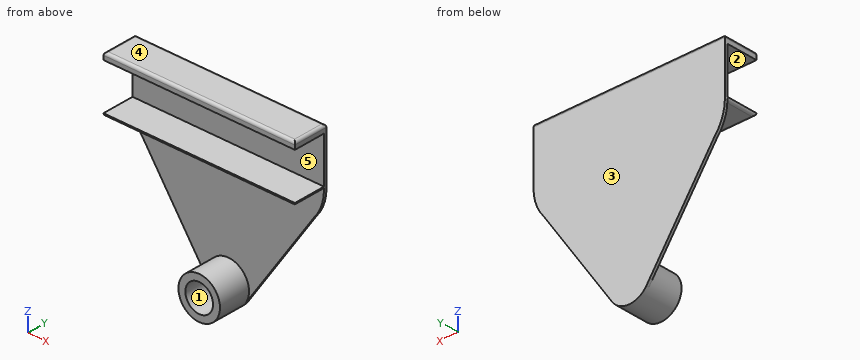
from build123d import *

# Parameters (mm, degrees)
F0_W     = 138.2855419193
F0_H     = 33
F0_R     = 10
F0_H_2   = 5
F0_H_3   = 2
F1_DEPTH = 2
F2_DEPTH = 25
F3_R     = 1.99999


# Not quite as in the source:
# - a fillet or chamfer is up to 0.001 mm smaller than in the source, because OpenCascade refuses the exact size


with BuildPart() as f1:
    # F0 (on Front) → F1 (new body)
    with BuildSketch(Plane.XZ):
        with BuildLine():
            ThreePointArc((61.670333147, -40.4906272888), (67.2163679442, -30.9053098713), (69.1427709597, -20))
            Line((69.1427709597, -20), (-69.1427709597, -20))
            ThreePointArc((-69.1427709597, -20), (-67.2163679442, -30.9053098713), (-61.670333147, -40.4906272888))
            Line((-61.670333147, -40.4906272888), (-12.4304277098, -113.3955027814))
            ThreePointArc((-12.4304277098, -113.3955027814), (-4.3899649403, -90.6567713599), (15, -105))
            ThreePointArc((15, -105), (14.3432286401, -109.3899649403), (12.4304277098, -113.3955027814))
            Line((12.4304277098, -113.3955027814), (61.670333147, -40.4906272888))
        make_face()
        with Locations((0, -1.5)):
            Rectangle(F0_W, F0_H)
        with BuildLine():
            ThreePointArc((-12.4304277098, -113.3955027814), (0, -120), (12.4304277098, -113.3955027814))
            ThreePointArc((12.4304277098, -113.3955027814), (14.3432286401, -109.3899649403), (15, -105))
            ThreePointArc((15, -105), (-4.3899649403, -90.6567713599), (-12.4304277098, -113.3955027814))
        make_face()
        with Locations((0, -105)):
            Circle(F0_R, mode=Mode.SUBTRACT)
        with Locations((0, 17.5)):
            Rectangle(F0_W, F0_H_2)
        with Locations((0, -105)):
            Circle(F0_R)
        with Locations((0, -19)):
            Rectangle(F0_W, F0_H_3)
    extrude(amount=F1_DEPTH)

    # F0 (on Front) → F2 (join)
    with BuildSketch(Plane.XZ):
        with Locations((0, 17.5)):
            Rectangle(F0_W, F0_H_2)
        with Locations((0, -19)):
            Rectangle(F0_W, F0_H_3)
        with BuildLine():
            ThreePointArc((-12.4304277098, -113.3955027814), (0, -120), (12.4304277098, -113.3955027814))
            ThreePointArc((12.4304277098, -113.3955027814), (14.3432286401, -109.3899649403), (15, -105))
            ThreePointArc((15, -105), (-4.3899649403, -90.6567713599), (-12.4304277098, -113.3955027814))
        make_face()
        with Locations((0, -105)):
            Circle(F0_R, mode=Mode.SUBTRACT)
    extrude(amount=F2_DEPTH)

    # F3 (radius 2 in the source; OpenCascade refuses exactly that, so slightly less here)
    f3_edges = [f1.edges().sort_by_distance(p)[0] for p in [
        (69.142771, -12.5, 20),
        (0, -25, 20),
        (-69.142771, -12.5, 20),
        (0, 0, 20),
        (0, -25, -20),
        (69.142771, -13.5, -20),
        (-69.142771, -13.5, -20),
    ]]
    fillet(f3_edges, radius=F3_R)


solid = f1.part
The model under review builds one solid part; all positions refer to its coordinate system, in mm. Face numbers are marked on the shaded views. A direction names the side the tool comes from. Round coordinates to 2 decimals unless told otherwise and drop trailing zeros. Write each loop counter-clockwise with the first axis right and the second up, starting at its lowest first coordinate (ties: lowest second). Pieces come first, ordered by that corner, then holes. Notation, with made-up numbers: (88, 51) -> (133, 51) arc R17 ccw to (133, 63) -> close; hole circle Ø9 at (56, 84.5). An arc over 180 degrees is marked (long way). Answer as a JSON object with one key per item and string values.
1. Machinability: for the marked faces 1 and 2, which of the approach directions +Z, -Z, +X, -X, +Y, -Y give a long, thin tool a straight path to every point of the face, cutting with its end or side? Answer none if there is none.
Results found:
{"face 1": "-Y", "face 2": "+X, -X, -Y"}
2. Clearance check with flat-ended pins moving along their axes: pin 1 (16.5 mm diameter, centred on x = 9, z = 0, fed in from -Y); pin 2 (10 mm diameter, centred on x = 5, z = -100.5, fed in from -Y); pin 3 (1 mm diameter, centred on y = -4.5, z = -17, fed in from -X); pin 4 (4 mm diameter, centred on x = 34, y = -4.5, fed in from -Z). State where each tip first meets the part, or that it passes through.
Results found:
{"pin 1": "stops at y = -2", "pin 2": "stops at y = -25", "pin 3": "passes through", "pin 4": "stops at z = -20"}
3. To check wall thickness, follow line 1 along Z through (x, y) = (41.5, -11.5); line 2 along X through (y, z) = (-18.25, -105); line 3 along Y through (x, z) = (-24.5, -65). State the ranges of each line that lie inside material, in increasing order.
Results found:
{"line 1": "z = -20 to -18, 15 to 20", "line 2": "x = -15 to -10, 10 to 15", "line 3": "y = -2 to 0"}
4. We need section A-A on y = -7.25. State how many separate pieces and enclosed holes the cut face has, and give its area (3 significant figures).
Results found:
{"separate pieces": "3", "enclosed holes": "1", "area": "1,360 mm^2"}
5. The part is to be moulded in two halves that separate along Z. For the marked faces 3, 4 and 5, say which applies: pulls with the +Z half, pulls with the -Z half, needs draft (parallel to the pull), parting line crosses it, or undercut.
Results found:
{"face 3": "needs draft", "face 4": "pulls with the +Z half", "face 5": "undercut"}
6. We need section C-C on z = 8. State the section outline as (x, y) points.
Results found:
{"outline": "(-69.14, -2) -> (69.14, -2) -> (69.14, 0) -> (-69.14, 0) -> close"}
